Design review of the part built by this model. Coordinates are the model's own, in mm. Round coordinates to 2 decimals unless told otherwise and drop trailing zeros. Write each loop counter-clockwise with the first axis right and the second up, starting at its lowest first coordinate (ties: lowest second). Pieces come first, ordered by that corner, then holes. Notation, with made-up numbers: (-23, 86) - (-14, 86) arc R11 cw to (-14, 93) - close; hole circle Ø8 at (-35.75, 64.5). An arc over 180 degrees is marked (long way). Use one line per item in the form item = value.
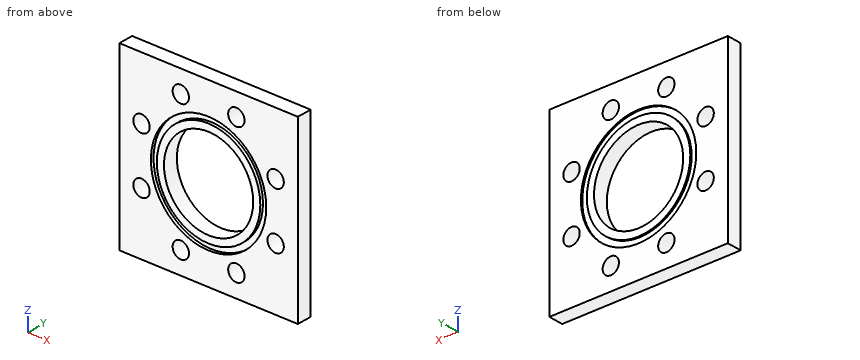
```python
from build123d import *

# Parameters (mm, degrees)
F0_W     = 76.2
F0_H     = 76.2
F1_DEPTH = 3.175
F2_R     = 3.4925
F3_DEPTH = 25.4
F4_R     = 19.05
F5_DEPTH = 25.4
F6_R     = 24.6253
F6_R_2   = 22.0853
F7_DEPTH = 1.3208
F8_R     = 24.6253
F8_R_2   = 22.0853
F9_DEPTH = 0.6604


with BuildPart() as f1:
    # F0 (on Front) → F1 (new body, symmetric)
    with BuildSketch(Plane.XZ):
        Rectangle(F0_W, F0_H)
    extrude(amount=F1_DEPTH, both=True)

    # F2 (on face) → F3 (cut)
    with BuildSketch(Plane.XZ.offset(3.175)):
        with Locations((11.8585942021, 28.6291789535)):
            Circle(F2_R)
        with Locations((-11.8585942021, 28.6291789535)):
            Circle(F2_R)
        with Locations((-28.6291789535, 11.8585942021)):
            Circle(F2_R)
        with Locations((-28.6291789535, -11.8585942021)):
            Circle(F2_R)
        with Locations((-11.8585942021, -28.6291789535)):
            Circle(F2_R)
        with Locations((11.8585942021, -28.6291789535)):
            Circle(F2_R)
        with Locations((28.6291789535, -11.8585942021)):
            Circle(F2_R)
        with Locations((28.6291789535, 11.8585942021)):
            Circle(F2_R)
    extrude(amount=-F3_DEPTH, mode=Mode.SUBTRACT)

    # F4 (on face) → F5 (cut)
    with BuildSketch(Plane.XZ.offset(3.175)):
        Circle(F4_R)
    extrude(amount=-F5_DEPTH, mode=Mode.SUBTRACT)

    # F6 (on face) → F7 (cut)
    with BuildSketch(Plane.XZ.offset(3.175)):
        Circle(F6_R)
        Circle(F6_R_2, mode=Mode.SUBTRACT)
    extrude(amount=-F7_DEPTH, mode=Mode.SUBTRACT)

    # F8 (on face) → F9 (cut)
    with BuildSketch(Plane(origin=(0, 3.175, 0), x_dir=(-1, 0, 0), z_dir=(0, 1, 0))):
        Circle(F8_R)
        Circle(F8_R_2, mode=Mode.SUBTRACT)
    extrude(amount=-F9_DEPTH, mode=Mode.SUBTRACT)


solid = f1.part
```
Q1. We need section D-D on x = -23.5. Write out the cut boundary in (y, z) (3 decimals), then the cut area to 3 significant figures.
Calculated:
outline = (-3.175, -38.1) - (3.175, -38.1) - (3.175, -7.359) - (2.515, -7.359) - (2.515, 7.359) - (3.175, 7.359) - (3.175, 38.1) - (-3.175, 38.1) - (-3.175, 7.359) - (-1.854, 7.359) - (-1.854, -7.359) - (-3.175, -7.359) - close
area = 455 mm2
Q2. We need section C-C on y = 1. State how many separate pieces and enclosed holes the cut face has, then the cut area to 3 significant figures.
Calculated:
separate_pieces = 1
enclosed_holes = 9
area = 4,360 mm2
Q3. We need section A-A on z = 0. Write out the cut boundary in (x, y) (3 decimals).
Calculated:
outline = (-38.1, -3.175) - (-24.625, -3.175) - (-24.625, -1.854) - (-22.085, -1.854) - (-22.085, -3.175) - (-19.05, -3.175) - (-19.05, 3.175) - (-22.085, 3.175) - (-22.085, 2.515) - (-24.625, 2.515) - (-24.625, 3.175) - (-38.1, 3.175) - close; (19.05, -3.175) - (22.085, -3.175) - (22.085, -1.854) - (24.625, -1.854) - (24.625, -3.175) - (38.1, -3.175) - (38.1, 3.175) - (24.625, 3.175) - (24.625, 2.515) - (22.085, 2.515) - (22.085, 3.175) - (19.05, 3.175) - close
Q4. We need section B-B on x = 0. Write out the cut boundary in (y, z) (3 decimals).
Calculated:
outline = (-3.175, -38.1) - (3.175, -38.1) - (3.175, -24.625) - (2.515, -24.625) - (2.515, -22.085) - (3.175, -22.085) - (3.175, -19.05) - (-3.175, -19.05) - (-3.175, -22.085) - (-1.854, -22.085) - (-1.854, -24.625) - (-3.175, -24.625) - close; (-3.175, 19.05) - (3.175, 19.05) - (3.175, 22.085) - (2.515, 22.085) - (2.515, 24.625) - (3.175, 24.625) - (3.175, 38.1) - (-3.175, 38.1) - (-3.175, 24.625) - (-1.854, 24.625) - (-1.854, 22.085) - (-3.175, 22.085) - close
Q5. For P1, Ø6.5, axis at x = -11.86, z = 28.63, coming from the +Y side (3 decimals); P2, Ø1, axis at x = -10.5, z = -20.5, coming from the +Y side, all flat-tipped, find the tip position at first contact; note any pin that passes through.
Calculated:
P1 = through
P2 = 2.51
Q6. To check wall thickness, follow line 1 along Z through (x, y) = (0, -2.8); line 2 along Z through (x, y) = (-13, -2); line 3 along Z through (x, y) = (0, 0.75). State the ranges of each line that lie inside material, in increasing order. Write a range as from..to.
Calculated:
line_1 = -38.1..-24.63, -22.09..-19.05, 19.05..22.09, 24.63..38.1
line_2 = -38.1..-31.93, -25.33..-20.91, -17.85..-13.92, 13.92..17.85, 20.91..25.33, 31.93..38.1
line_3 = -38.1..-19.05, 19.05..38.1
